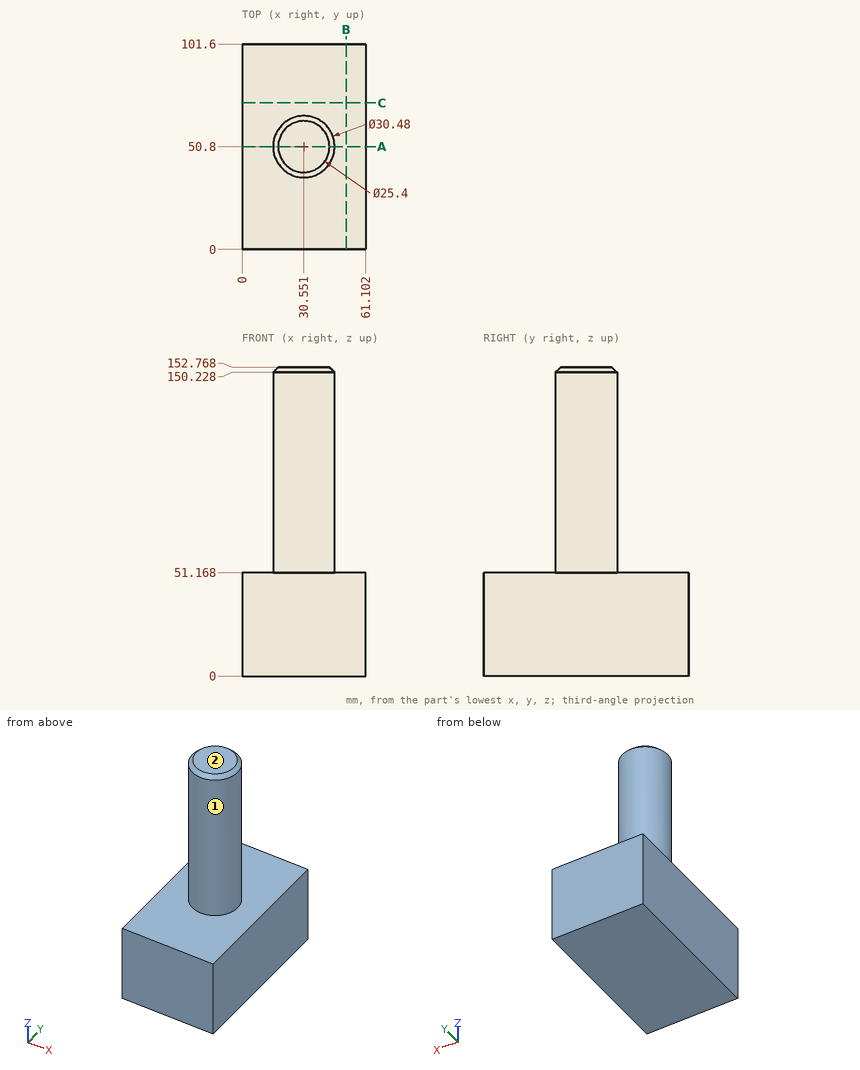
Can you work these out from the drawing? Everything is in mm from the part's minimum corner. A direction names the side the tool comes from. Coordinates: 2 decimals unless noted, no trailing zeros. Loops run counter-clockwise (first coordinate to the right, second up) from the corner with the lowest first, then second, coordinate; pieces in that order, holes last.
1) Will these pins go through, and if not, where does the flat tip stop? pin 1 Ø8 at (x, z) = (19.5, 125.5) entering from -Y; pin 2 Ø3 at (y, z) = (52, 107.5) entering from +X; pin 3 Ø12 at (x, y) = (43.5, 40) entering from -Z; pin 4 Ø2 at (x, y) = (51, 63) entering from +Z.
Reported:
pin 1: stops at y = 37.29
pin 2: stops at x = 45.79
pin 3: stops at z = 0
pin 4: stops at z = 51.17
2) Please list where these lines run through material, in increasing order: line 1 along Z through (x, y) = (12.5, 13); line 2 along X through (y, z) = (51, 77); line 3 along Y through (x, z) = (33.5, 142).
Reported:
line 1: z = 0 to 51.17
line 2: x = 15.31 to 45.79
line 3: y = 35.85 to 65.75
3) Which directions (+Z, -Z, +X, -X, +Y, -Y) give clear straight access to the entire face, cutting with the end or side of a thin tool? Please do the marked faces 1 and 2.
Reported:
face 1: +Z
face 2: +Z, +X, -X, +Y, -Y
4) Imagine slicing it at B-B (x = 51.5). List the corners of the cut face in (y, z) for me.
Reported:
outline: (0, 0) - (101.6, 0) - (101.6, 51.17) - (0, 51.17) - close
5) Imagine slicing it at C-C (y = 72.5). List the corners of the cut face in (x, z) for me, and give its area (3 significant figures).
Reported:
outline: (0, 0) - (61.1, 0) - (61.1, 51.17) - (0, 51.17) - close
area: 3,130 mm2
6) Imagine slicing it at A-A (y = 50.8). List the corners of the cut face in (x, z) for me, and give its area (3 significant figures).
Reported:
outline: (0, 0) - (61.1, 0) - (61.1, 51.17) - (45.79, 51.17) - (45.79, 150.23) - (43.25, 152.77) - (17.85, 152.77) - (15.31, 150.23) - (15.31, 51.17) - (0, 51.17) - close
area: 6,220 mm2
